```python
from build123d import *

# Parameters (mm, degrees)
F1_DEPTH = 2.5
F2_W     = 35
F2_H     = 2
F3_DEPTH = 4
F4_W     = 50
F4_H     = 0.5
F5_DEPTH = 3


with BuildPart() as f1:
    # F0 (on Top) → F1 (new body)
    with BuildSketch(Plane.XY):
        Polygon((-14.433757, -25), (14.433757, -25), (28.867513, 0), (14.433757, 25), (-14.433757, 25), (-28.867513, 0), align=None)
    extrude(amount=F1_DEPTH)

    # F2 (on face) → F3 (join)
    with BuildSketch(Plane.XY.offset(2.5)):
        Rectangle(F2_W, F2_H)
    extrude(amount=F3_DEPTH)

    # F4 (on face) → F5 (cut)
    with BuildSketch(Plane.XY.offset(6.5)):
        with Locations((0.279709, 0)):
            Rectangle(F4_W, F4_H)
    extrude(amount=-F5_DEPTH, mode=Mode.SUBTRACT)


solid = f1.part
```
Verification items for the finished model (mm, model axes). A direction names the side the tool comes from. Give positions to 0.01 mm unless a question says otherwise; leave off trailing zeros. Write each loop counter-clockwise with the first axis right and the second up, starting at its lowest first coordinate (ties: lowest second). Pieces come first, ordered by that corner, then holes. Notation, with made-up numbers: M 82.5,37.25 L 131.5,37.25 A15 cw 131.5,54.25 Z; hole C 42,56 d10. An arc over 180 degrees is marked long. One line per question, with ' | ' between items.
1) Section check C-C on z = 0.75. Enter the section's corners in (x, y), plus the area to 3 significant figures.
Result:
outline: M -28.87,0 L -14.43,-25 L 14.43,-25 L 28.87,0 L 14.43,25 L -14.43,25 Z | area: 2,170 mm2
2) Set-up check for faces 4 (the flat face through (0, -0.25, 5)), 5 (the flat face through (0, -1, 4)), 6 (the flat face through (-17.5, -0.5, 4.5)), 7 (the flat face through (17.5, -0.5, 4.5)), 8 (the flat face through (0, 1, 4)): record each of +Z, -Z, +X, -X, +Y, -Y from which the full face is reachable in a straight line by a thin tool's end or side.
Result:
face 4: +Z, +X, -X | face 5: +Z, +X, -X, -Y | face 6: +Z, -X, +Y, -Y | face 7: +Z, +X, +Y, -Y | face 8: +Z, +X, -X, +Y
3) Thickness scan on line 1 along Y through (x, z) = (12.5, 4.5); line 2 along Z through (x, y) = (4.5, -14.5); line 3 along X through (y, z) = (0.5, 4.75). Record the ranges inside material, lowest first. Write a range as [from, to].
Result:
line 1: y = [-1, -0.25], [0.25, 1] | line 2: z = [0, 2.5] | line 3: x = [-17.5, 17.5]
4) Section check B-B on x = -9.5. Enter the section's corners in (y, z), plus the area to 4 significant figures.
Result:
outline: M -25,0 L 25,0 L 25,2.5 L 1,2.5 L 1,6.5 L 0.25,6.5 L 0.25,3.5 L -0.25,3.5 L -0.25,6.5 L -1,6.5 L -1,2.5 L -25,2.5 Z | area: 131.5 mm2
5) Mould release check, pull along Y, two halves, no side actions. Record for faces 1 (the flat face through (0, 0, 0)), 2 (the flat face through (0, 0.25, 5)), 3 (the flat face through (-21.55, 12.675, 1.232)): released by +Y, released by -Y, zero draft, split by the parting line, or undercut.
Result:
face 1: zero draft | face 2: undercut | face 3: released by +Y
6) Section check A-A on z = 4.25. Enter the section's corners in (x, y), plus the area to 3 significant figures.
Result:
outline: M -17.5,-1 L 17.5,-1 L 17.5,-0.25 L -17.5,-0.25 Z; M -17.5,0.25 L 17.5,0.25 L 17.5,1 L -17.5,1 Z | area: 52.5 mm2
7) Gauge pin test, flat ends, axial feed: pin 1 Ø0.9 at (x, z) = (2, 5.5) entering from -Y; pin 2 Ø2 at (y, z) = (18, 3) entering from +X; pin 3 Ø2 at (x, z) = (-6, 5.5) entering from +Y. Record the tip position at first contact, or that the pin passes through.
Result:
pin 1: stops at y = -1 | pin 2: stops at x = 18.98 | pin 3: stops at y = 1
8) Section check D-D on y = -3. Enter the section's corners in (x, z), plus the area to 3 significant figures.
Result:
outline: M -27.14,0 L 27.14,0 L 27.14,2.5 L -27.14,2.5 Z | area: 136 mm2
